Verification items for the finished model (mm, model axes). A direction names the side the tool comes from. Round coordinates to 2 decimals unless told otherwise and drop trailing zeros. Write each loop counter-clockwise with the first axis right and the second up, starting at its lowest first coordinate (ties: lowest second). Pieces come first, ordered by that corner, then holes. Notation, with made-up numbers: M -19.75,5.25 L -11.75,5.25 A19 cw -11.75,40.25 Z; hole C 51,36.25 d9. An arc over 180 degrees is marked long. One line per question, with ' | ' between items. Start each with the question number.
Q1. Cross-section at D-D (y = 1.2). State how many separate pieces and enclosed holes the cut face has, then the cut area to 3 significant figures.
Q2. Release check for a two-part mould opening along X. For faces 1 (the face through (7, 2, 36.16)), 2 (the face through (21.44, 2.03, 18.99)), 3 (the face through (-9.672, 2.028, -1.137)), 4 (the face through (-18, 2, -5)) record: released by +X, released by -X, zero draft, split by the parting line, or undercut.
Q3. Thickness scan on line 1 along X through (y, z) = (2.8, 41.66); line 2 along X through (y, z) = (3.5, 16.5); line 3 along X through (y, z) = (3, -24.5). Record the ranges inside material, lowest first. Write a range as from..to.
Q4. Tool access check on faces 5 (the face through (4, 2, 38)), 6 (the face through (-5, 2, -24)), 7 (the face through (-11.226, 2.028, 24.307)). Record the directions out of +Z, -Z, +X, -X, +Y, -Y that give a thin tool (end or side, any length) a straight path to the whole face; none if there is none.
Q5. Cross-section at C-C (z = 29.5). Record the boundary of the cut face in (x, y), then the cut area to 3 significant figures.
Q6. Cross-section at A-A (x = 30). Record the boundary of the cut face in (y, z).
Q7. Cross-section at B-B (z = 41.66). Record the boundary of the cut face in (x, y), then the cut area to 3 significant figures.
Q8. Gauge pin test, flat ends, axial feed: pin 1 (1.8 mm diameter, centred on x = -30, z = 41.66, fed in from -Y); pin 2 (1.2 mm diameter, centred on x = -18, y = 2.5, fed in from -Z); pin 3 (2 mm diameter, centred on x = 11, y = 1.5, fed in from -Z); pin 4 (2 mm diameter, centred on y = 1.5, z = -26, fed in from -X). Record the tip position at first contact, or that the pin passes through.
from build123d import *

# Parameters (mm, degrees)
ESQUISSE1_R             = 1.5
ESQUISSE1_W             = 4
ESQUISSE1_H             = 7
ESQUISSE1_W_2           = 6
ESQUISSE1_H_2           = 4
BOSS_EXTRU_1_DEPTH      = 4
ENL_V_MAT_EXTRU_1_REACH = 59.99
ENL_V_MAT_EXTRU_2_REACH = 59.99
ENL_V_MAT_EXTRU_3_REACH = 59.99
CONG_1_R                = 3.5
CONG_2_R                = 3.5
CONG_3_R                = 1.5
ENL_V_MAT_EXTRU_4_REACH = 59.99
CONG_4_R                = 3
CONG_5_R                = 3
ENL_V_MAT_EXTRU_5_REACH = 59.99
ESQUISSE8_R             = 3.5
CONG_6_R                = 1.5


with BuildPart() as part:
    # Esquisse1 → Boss.-Extru.1 (new body)
    with BuildSketch(Plane(origin=(0, 0, 0), x_dir=(1, 0, 0), z_dir=(0, 1, 0))):
        Polygon((-20.28, 5), (-22.28, 5), (-22.28, -37), (-34.66, -37), (-34.66, -46.32), (34.66, -46.32), (34.66, -37), (22.28, -37), (22.28, 5), (20.28, 5), (16.28, 5), (16.28, 13), (5, 13), (5, 35), (-5, 35), (-5, 13), (-16.28, 13), (-16.28, 5), align=None)
        with Locations(Location((-5, 0, 0), (0, 0, 270))):
            Circle(ESQUISSE1_R, mode=Mode.SUBTRACT)
        with Locations(Location((5, 0, 0), (0, 0, 90))):
            Circle(ESQUISSE1_R, mode=Mode.SUBTRACT)
        with Locations(Location((-30, -41.66, 0), (0, 0, 270))):
            Circle(ESQUISSE1_R, mode=Mode.SUBTRACT)
        with Locations(Location((30, -41.66, 0), (0, 0, 90))):
            Circle(ESQUISSE1_R, mode=Mode.SUBTRACT)
        with Locations((0, 27.42)):
            Rectangle(ESQUISSE1_W, ESQUISSE1_H, mode=Mode.SUBTRACT)
        with Locations((-17.5, -13.5)):
            Rectangle(ESQUISSE1_W, ESQUISSE1_H, mode=Mode.SUBTRACT)
        with Locations((-7, -38.16)):
            Rectangle(ESQUISSE1_W_2, ESQUISSE1_H_2, mode=Mode.SUBTRACT)
        with Locations((7, -38.16)):
            Rectangle(ESQUISSE1_W_2, ESQUISSE1_H_2, mode=Mode.SUBTRACT)
        with Locations((17.5, -13.5)):
            Rectangle(ESQUISSE1_W, ESQUISSE1_H, mode=Mode.SUBTRACT)
    extrude(amount=BOSS_EXTRU_1_DEPTH)

    # Esquisse2 → Enlèv. mat.-Extru.1 (cut, up to next)
    with BuildSketch(Plane(origin=(0, 4, 0), x_dir=(1, 0, 0), z_dir=(0, 1, 0)), mode=Mode.PRIVATE) as enl_v_mat_extru_1_sk1:
        with BuildLine():
            ThreePointArc((-14.9974668, -7.843519448), (-14.058937243, -8.627559279), (-13.321584394, -9.603195975))
            ThreePointArc((-13.321584394, -9.603195975), (-12.428040198, -10.235555734), (-11.361521034, -9.988904221))
            ThreePointArc((-11.361521034, -9.988904221), (-8.447920047, -8.097394436), (-5.290042477, -6.650090308))
            ThreePointArc((-5.290042477, -6.650090308), (-4.088898303, -4.755535803), (-5.589901119, -3.088480121))
            ThreePointArc((-5.589901119, -3.088480121), (-7.276914991, -2.168490468), (-8.113566287, -0.438631695))
            ThreePointArc((-8.113566287, -0.438631695), (-9.70546362, 1.141857781), (-11.656322949, 0.034504187))
            ThreePointArc((-11.656322949, 0.034504187), (-13.25585737, -3.049060247), (-15.287160414, -5.866982872))
            ThreePointArc((-15.287160414, -5.866982872), (-15.585513038, -6.920209252), (-14.9974668, -7.843519448))
        make_face()
    enl_v_mat_extru_1_tool1 = extrude(enl_v_mat_extru_1_sk1.sketch, amount=-ENL_V_MAT_EXTRU_1_REACH, mode=Mode.PRIVATE) & part.part
    # Esquisse2 → Enlèv. mat.-Extru.1 (cut, up to next)
    with BuildSketch(Plane(origin=(0, 4, 0), x_dir=(1, 0, 0), z_dir=(0, 1, 0)), mode=Mode.PRIVATE) as enl_v_mat_extru_1_sk2:
        with BuildLine():
            ThreePointArc((5.589901119, -3.088480121), (4.088898303, -4.755535803), (5.290042477, -6.650090308))
            ThreePointArc((5.290042477, -6.650090308), (8.447920047, -8.097394436), (11.361521034, -9.988904221))
            ThreePointArc((11.361521034, -9.988904221), (12.428040198, -10.235555734), (13.321584394, -9.603195975))
            ThreePointArc((13.321584394, -9.603195975), (14.058937243, -8.627559279), (14.9974668, -7.843519448))
            ThreePointArc((14.9974668, -7.843519448), (15.585513038, -6.920209252), (15.287160414, -5.866982872))
            ThreePointArc((15.287160414, -5.866982872), (13.25585737, -3.049060247), (11.656322949, 0.034504187))
            ThreePointArc((11.656322949, 0.034504187), (9.70546362, 1.141857781), (8.113566287, -0.438631695))
            ThreePointArc((8.113566287, -0.438631695), (7.276914991, -2.168490468), (5.589901119, -3.088480121))
        make_face()
    enl_v_mat_extru_1_tool2 = extrude(enl_v_mat_extru_1_sk2.sketch, amount=-ENL_V_MAT_EXTRU_1_REACH, mode=Mode.PRIVATE) & part.part
    add(enl_v_mat_extru_1_tool1.solids().sort_by_distance((-10.104676, 4, 4.861596))[0], mode=Mode.SUBTRACT)
    add(enl_v_mat_extru_1_tool2.solids().sort_by_distance((10.104676, 4, 4.861596))[0], mode=Mode.SUBTRACT)

    # Esquisse3 → Enlèv. mat.-Extru.2 (cut, up to next)
    with BuildSketch(Plane(origin=(0, 4, 0), x_dir=(1, 0, 0), z_dir=(0, 1, 0)), mode=Mode.PRIVATE) as enl_v_mat_extru_2_sk1:
        with BuildLine():
            ThreePointArc((-3.934570919, -34.661427668), (-3.25, -34.860961894), (-2.734912831, -35.354050587))
            ThreePointArc((-2.734912831, -35.354050587), (-1.93927123, -36.028172694), (-0.901821799, -36.133931151))
            ThreePointArc((-0.901821799, -36.133931151), (0, -36.043871504), (0.901821799, -36.133931151))
            ThreePointArc((0.901821799, -36.133931151), (1.93927123, -36.028172694), (2.734912831, -35.354050587))
            ThreePointArc((2.734912831, -35.354050587), (3.25, -34.860961894), (3.934570919, -34.661427668))
            ThreePointArc((3.934570919, -34.661427668), (7.745022524, -30.318334752), (3.241418184, -26.699005331))
            ThreePointArc((3.241418184, -26.699005331), (0, -26.910051622), (-3.241418184, -26.699005331))
            ThreePointArc((-3.241418184, -26.699005331), (-7.745022524, -30.318334752), (-3.934570919, -34.661427668))
        make_face()
    enl_v_mat_extru_2_tool1 = extrude(enl_v_mat_extru_2_sk1.sketch, amount=-ENL_V_MAT_EXTRU_2_REACH, mode=Mode.PRIVATE) & part.part
    add(enl_v_mat_extru_2_tool1.solids().sort_by_distance((0, 4, 31.014631))[0], mode=Mode.SUBTRACT)

    # Esquisse4 → Enlèv. mat.-Extru.3 (cut, up to next)
    with BuildSketch(Plane(origin=(0, 4, 0), x_dir=(1, 0, 0), z_dir=(0, 1, 0)), mode=Mode.PRIVATE) as enl_v_mat_extru_3_sk1:
        with BuildLine():
            ThreePointArc((-3.204236741, -23.492683837), (0, -23.72926901), (3.204236741, -23.492683837))
            ThreePointArc((3.204236741, -23.492683837), (3.729211384, -23.484474006), (4.238200501, -23.613298912))
            ThreePointArc((4.238200501, -23.613298912), (5.947114761, -23.612368685), (7.184676805, -22.433882792))
            ThreePointArc((7.184676805, -22.433882792), (7.833923694, -20.976940348), (8.452629907, -19.506768443))
            ThreePointArc((8.452629907, -19.506768443), (8.650133896, -14.04633429), (5.268411363, -9.754562897))
            ThreePointArc((5.268411363, -9.754562897), (4.141434744, -9.367776338), (2.957336552, -9.500409716))
            ThreePointArc((2.957336552, -9.500409716), (0, -9.996838884), (-2.957336552, -9.500409716))
            ThreePointArc((-2.957336552, -9.500409716), (-4.141434744, -9.367776338), (-5.268411363, -9.754562897))
            ThreePointArc((-5.268411363, -9.754562897), (-8.650133896, -14.04633429), (-8.452629907, -19.506768443))
            ThreePointArc((-8.452629907, -19.506768443), (-7.833923694, -20.976940348), (-7.184676805, -22.433882792))
            ThreePointArc((-7.184676805, -22.433882792), (-5.947114761, -23.612368685), (-4.238200501, -23.613298912))
            ThreePointArc((-4.238200501, -23.613298912), (-3.729211384, -23.484474006), (-3.204236741, -23.492683837))
        make_face()
    enl_v_mat_extru_3_tool1 = extrude(enl_v_mat_extru_3_sk1.sketch, amount=-ENL_V_MAT_EXTRU_3_REACH, mode=Mode.PRIVATE) & part.part
    add(enl_v_mat_extru_3_tool1.solids().sort_by_distance((0, 4, 16.711487))[0], mode=Mode.SUBTRACT)

    # Congé1
    cong_1_edges = [part.edges().sort_by_distance(p)[0] for p in [
        (-5, 2, -35),
        (5, 2, -35),
    ]]
    fillet(cong_1_edges, radius=CONG_1_R)

    # Congé2
    cong_2_edges = [part.edges().sort_by_distance(p)[0] for p in [
        (-5, 2, -13),
        (5, 2, -13),
    ]]
    fillet(cong_2_edges, radius=CONG_2_R)

    # Congé3
    cong_3_edges = [part.edges().sort_by_distance(p)[0] for p in [
        (22.28, 2, -5),
        (-22.28, 2, -5),
        (-16.28, 2, -13),
        (16.28, 2, -13),
    ]]
    fillet(cong_3_edges, radius=CONG_3_R)

    # Esquisse7 → Enlèv. mat.-Extru.4 (cut, up to next)
    with BuildSketch(Plane(origin=(0, 4, 0), x_dir=(1, 0, 0), z_dir=(0, 1, 0)), mode=Mode.PRIVATE) as enl_v_mat_extru_4_sk1:
        with BuildLine():
            Line((-22.28, -17), (-22.28, -37))
            ThreePointArc((-22.28, -37), (-16.000012961, -35.267986448), (-11.495708343, -30.561677059))
            ThreePointArc((-11.495708343, -30.561677059), (-11.263143502, -24.222708134), (-16.146891575, -20.174792843))
            ThreePointArc((-16.146891575, -20.174792843), (-17.81186512, -19.879037913), (-19.5, -19.78))
            ThreePointArc((-19.5, -19.78), (-21.465756852, -18.965756852), (-22.28, -17))
        make_face()
    enl_v_mat_extru_4_tool1 = extrude(enl_v_mat_extru_4_sk1.sketch, amount=-ENL_V_MAT_EXTRU_4_REACH, mode=Mode.PRIVATE) & part.part
    enl_v_mat_extru_4 = enl_v_mat_extru_4_tool1.solids().sort_by_distance((-17.328715, 4, 27.806477))[0]
    add(enl_v_mat_extru_4, mode=Mode.SUBTRACT)

    # Symétrie1: Enlèv. mat.-Extru.4 across plane
    add(enl_v_mat_extru_4.mirror(Plane(origin=(0, 0, 0), x_dir=(0, 0, 1), z_dir=(1, 0, 0))), mode=Mode.SUBTRACT)

    # Congé4
    cong_4_edges = [part.edges().sort_by_distance(p)[0] for p in [
        (-34.66, 2, 46.32),
        (-34.66, 2, 37),
    ]]
    fillet(cong_4_edges, radius=CONG_4_R)

    # Congé5
    cong_5_edges = [part.edges().sort_by_distance(p)[0] for p in [
        (34.66, 2, 37),
        (34.66, 2, 46.32),
    ]]
    fillet(cong_5_edges, radius=CONG_5_R)

    # Esquisse8 → Enlèv. mat.-Extru.5 (cut, up to next)
    with BuildSketch(Plane(origin=(0, 4, 0), x_dir=(1, 0, 0), z_dir=(0, 1, 0)), mode=Mode.PRIVATE) as enl_v_mat_extru_5_sk1:
        with Locations((-15, -46.32)):
            Circle(ESQUISSE8_R)
    enl_v_mat_extru_5_tool1 = extrude(enl_v_mat_extru_5_sk1.sketch, amount=-ENL_V_MAT_EXTRU_5_REACH, mode=Mode.PRIVATE) & part.part
    # Esquisse8 → Enlèv. mat.-Extru.5 (cut, up to next)
    with BuildSketch(Plane(origin=(0, 4, 0), x_dir=(1, 0, 0), z_dir=(0, 1, 0)), mode=Mode.PRIVATE) as enl_v_mat_extru_5_sk2:
        with Locations((15, -46.32)):
            Circle(ESQUISSE8_R)
    enl_v_mat_extru_5_tool2 = extrude(enl_v_mat_extru_5_sk2.sketch, amount=-ENL_V_MAT_EXTRU_5_REACH, mode=Mode.PRIVATE) & part.part
    add(enl_v_mat_extru_5_tool1.solids().sort_by_distance((-15, 4, 46.32))[0], mode=Mode.SUBTRACT)
    add(enl_v_mat_extru_5_tool2.solids().sort_by_distance((15, 4, 46.32))[0], mode=Mode.SUBTRACT)

    # Congé6
    cong_6_edges = [part.edges().sort_by_distance(p)[0] for p in [
        (-18.5, 2, 46.32),
        (-11.5, 2, 46.32),
        (11.5, 2, 46.32),
        (18.5, 2, 46.32),
    ]]
    fillet(cong_6_edges, radius=CONG_6_R)


solid = part.part
Determined:
1) separate pieces: 1 | enclosed holes: 13 | area: 1,970 mm²
2) face 1: undercut | face 2: released by +X | face 3: undercut | face 4: zero draft
3) line 1: x = -34.66..-31.5, -28.5..28.5, 31.5..34.66 | line 2: x = -22.28..-19.5, -15.5..-9.04, 9.04..15.5, 19.5..22.28 | line 3: x = -5..-2, 2..5
4) face 5: +Y, -Y | face 6: -Z, -X, +Y, -Y | face 7: -X, +Y, -Y
5) outline: M -11.03,0 L -7.59,0 L -7.59,4 L -11.03,4 Z; M 7.59,0 L 11.03,0 L 11.03,4 L 7.59,4 Z | area: 27.5 mm²
6) outline: M 0,37 L 4,37 L 4,40.16 L 0,40.16 Z; M 0,43.16 L 4,43.16 L 4,46.32 L 0,46.32 Z
7) outline: M -34.66,0 L -31.5,0 L -31.5,4 L -34.66,4 Z; M -28.5,0 L 28.5,0 L 28.5,4 L -28.5,4 Z; M 31.5,0 L 34.66,0 L 34.66,4 L 31.5,4 Z | area: 253 mm²
8) pin 1: passes through | pin 2: stops at z = -5 | pin 3: stops at z = -13 | pin 4: stops at x = -5
